Autodesk Inventor part; units mm, degrees
ref_plane "YZ Plane" through (0, 0, 0) normal (1, 0, 0) x (0, 1, 0)
ref_plane "XZ Plane" through (0, 0, 0) normal (0, 1, 0) x (-1, 0, 0)
ref_plane "XY Plane" through (0, 0, 0) normal (0, 0, 1) x (1, 0, 0)
sketch "Sketch1" plane through (0, 0, 0) normal (0, 1, 0) x (-1, 0, 0)
  point P0 (0, 0)
sketch "Sketch2" plane through (0, 0, 0) normal (0, 1, 0) x (-1, 0, 0)
  line L0 (0, 0) -> (10, 0)
  line L1 (10, 0) -> (10, -5)
  line L2 (10, -5) -> (0, -5)
  line L3 (0, -5) -> (0, 0)
  dimension "d0" = 10
  dimension "d1" = 5
extrude "Extrusion1" add sketch "Sketch2" along normal blind 3
sketch "Sketch3" plane through (0, 3, 0) normal (0, 1, 0) x (1, 0, 0)
  line L0 (-10, 5) -> (-10, 0)
  line L1 (-10, 2.5) -> (0, 2.5)
  line L2 (-10, 2.5) -> (-8.5, 2.5)
  line L3 (0, 2.5) -> (-1.5, 2.5)
  circle A0 centre (-8.5, 2.5) radius 1.5
  circle A1 centre (-1.5, 2.5) radius 1.5
  line L4 (0, 0) -> (0, 5)
  line L5 (-7.382, 1.5) -> (-2.618, 1.5)
  line L6 (-2.618, 3.5) -> (-7.382, 3.5)
extrude "Extrusion2" add sketch "Sketch3" along normal blind 4
sketch "Sketch4" plane through (0, 7, 0) normal (0, 1, 0) x (1, 0, 0)
  arc A0 (-10, 2.5) -> (-7.382, 1.5) centre (-8.5, 2.5) ccw
  circle A1 centre (-8.5, 2.5) radius 1.25
  arc A2 (-2.618, 1.5) -> (-2.618, 3.5) centre (-1.5, 2.5) ccw
  circle A3 centre (-1.5, 2.5) radius 1.25
  arc A4 (-2.618, 3.5) -> (-2.618, 1.5) centre (-1.5, 2.5) ccw
  arc A5 (-7.382, 1.5) -> (-7.382, 3.5) centre (-8.5, 2.5) ccw
  line L0 (-7.382, 1.5) -> (-2.618, 1.5)
  line L1 (-7.382, 3.5) -> (-2.618, 3.5)
  point P0 (0, 0)
extrude "Extrusion3" cut sketch "Sketch4" against normal blind 1 contours A1 | L0 A5 L1 A4 | A3
sketch "Sketch5" plane through (0, 0, 0) normal (0, -1, 0) x (1, 0, 0)
  line L0 (0, -5) -> (-10, -5)
  line L1 (0, -5) -> (-2, -5)
  line L2 (-10, -5) -> (-8, -5)
  line L3 (-2, -5) -> (-1.5, -5)
  line L4 (-1.5, -5) -> (-1.5, -5.5)
  line L5 (-2.5, -5.5) -> (-2.5, -5)
  line L6 (-2.5, -5) -> (-2, -5)
  line L7 (-8, -5) -> (-8.5, -5)
  line L8 (-8.5, -5) -> (-8.5, -5.5)
  line L9 (-7.5, -5.5) -> (-7.5, -5)
  line L10 (-7.5, -5) -> (-8, -5)
  arc A0 (-2.5, -5.5) -> (-1.5, -5.5) centre (-2, -5.5) ccw
  arc A1 (-8.5, -5.5) -> (-7.5, -5.5) centre (-8, -5.5) ccw
  point P0 (0, 0)
  dimension "d19" = 2
extrude "Extrusion4" add sketch "Sketch5" against normal blind 0.3
sketch "Sketch6" plane through (0, 0.3, 0) normal (0, 1, 0) x (1, 0, 0)
  arc A0 (-1.5, 5.5) -> (-2.5, 5.5) centre (-2, 5.5) ccw
  circle A1 centre (-2, 5.5) radius 0.4
  arc A2 (-7.5, 5.5) -> (-8.5, 5.5) centre (-8, 5.5) ccw
  circle A3 centre (-8, 5.5) radius 0.4
  point P0 (0, 0)
  dimension "d30" = 0.8
  dimension "d31" = 0.8
extrude "Extrusion5" cut sketch "Sketch6" against normal blind 0.3
thread "Thread1"
thread "Thread2"
properties part number "distanceSensor"
Input: part model. Units: mm. Frame: model coordinates. A direction names the side the tool comes from. Round coordinates to 2 decimals unless told otherwise and drop trailing zeros. Order: outer loops, then holes, each group sorted by start corner. A loop starts at its lowest first (then second) coordinate and runs counter-clockwise, first axis right, second up. Notation, with made-up numbers: (51, -30) - (88, -30) arc R29 ccw to (88, 3) - close; hole circle Ø6 at (40, 25). An arc over 180 degrees is marked (long way). Answer as a JSON object with one key per item and string values. Group by question number.
(1) Reachability of faces 1 (the face through (0, 1, -3)), 2 (the face through (-5, 3, -1)), 3 (the face through (-9, 6, -3)), 4 (the face through (-5, 3, -4)) from +Z, -Z, +X, -X, +Y, -Y: full face, straight path, thin tool, end or side. Return the list, or none.
(2) Material intervals for probe 1 along X at (y, z) = (6.45, -2.5); probe 2 along Z at (x, y) = (-8.5, 6.3); probe 3 along Y at (x, z) = (-3.25, -1.95), sorted ascending. Write a range as from..to.
(3) Cut plane A-A (y = 6.5). Return loops of the section in (x, z).
(4) Draft query along X for faces 5 (the face through (-10, 4.97, -2.45)), 6 (the face through (-10, 1, -2)), 7 (the face through (-5, 0, -3)). Return one class per face: released by +X, released by -X, zero draft, split by the parting line, or undercut.
(5) Pin query (flat end, axial travel): P1, Ø1.2, axis at x = -1.5, z = -2.5, coming from the +Y side; P2, Ø2.5, axis at x = -4, y = 4.5, coming from the +Z side; P3, Ø3.5, axis at x = -5, y = 4, coming from the -Z side. Return the tip coordinate at first contact, or that it passes through.
(6) Cut plane C-C (z = -2.1). Return loops of the section in (x, y), then the cut area to 3 significant figures.
(7) Cut plane B-B (x = -5). Return loops of the section in (y, z), then the cut area to 3 significant figures.
(8) Cut plane D-D (x = -2). Return loops of the section in (y, z), then the cut area to 3 significant figures.
Here are the results:
{
 "1": {"face 1": "+Z, -Z, +X, +Y, -Y", "face 2": "+Z, +Y", "face 3": "+Y", "face 4": "-Z, +Y"},
 "2": {"probe 1": "x = -10..-9.75, -7.25..-7, -3..-2.75, -0.25..0", "probe 2": "z = -4..-3.75, -1.25..-1", "probe 3": "y = 0..6"},
 "3": {"outline": "circle Ø3 at (-8.5, -2.5); circle Ø3 at (-1.5, -2.5); hole circle Ø2.5 at (-8.5, -2.5); hole circle Ø2.5 at (-1.5, -2.5)"},
 "4": {"face 5": "undercut", "face 6": "released by -X", "face 7": "zero draft"},
 "5": {"P1": "stops at y = 6", "P2": "stops at z = -1.5", "P3": "stops at z = -5"},
 "6": {"outline": "(-10, 0) - (0, 0) - (0, 3) - (-0.05, 3) - (-0.05, 7) - (-0.32, 7) - (-0.32, 6) - (-2.68, 6) - (-2.68, 7) - (-2.95, 7) - (-2.95, 6) - (-7.05, 6) - (-7.05, 7) - (-7.32, 7) - (-7.32, 6) - (-9.68, 6) - (-9.68, 7) - (-9.95, 7) - (-9.95, 3) - (-10, 3) - close", "area": "60.7 mm^2"},
 "7": {"outline": "(0, -5) - (3, -5) - (3, -3.5) - (6, -3.5) - (6, -1.5) - (3, -1.5) - (3, 0) - (0, 0) - close", "area": "21.0 mm^2"},
 "8": {"outline": "(0, -6) - (0.3, -6) - (0.3, -5.9) - (0, -5.9) - close; (0, -5.1) - (0.3, -5.1) - (0.3, -5) - (3, -5) - (3, -3.91) - (7, -3.91) - (7, -3.65) - (6, -3.65) - (6, -1.35) - (7, -1.35) - (7, -1.09) - (3, -1.09) - (3, 0) - (0, 0) - close", "area": "24.1 mm^2"}
}
